Here's how the part is built. I have some questions about the finished solid (model axes, mm). Give positions to 0.01 mm unless a question says otherwise; leave off trailing zeros. Order: outer loops, then holes, each group sorted by start corner. A loop starts at its lowest first (then second) coordinate and runs counter-clockwise, first axis right, second up.
from build123d import *

# Parameters (mm, degrees)
SKETCH1_R           = 4.5
BOSS_EXTRUDE1_DEPTH = 3
SKETCH3_R           = 1.5
CUT_EXTRUDE1_DEPTH  = 10


with BuildPart() as part:
    # Sketch1 → Boss-Extrude1 (new body)
    with BuildSketch(Plane(origin=(0, 0, 0), x_dir=(0, 0, -1), z_dir=(1, 0, 0))):
        with BuildLine():
            Line((0.169822647, 50), (0.169822647, -50))
            ThreePointArc((0.169822647, -50), (-14.830177353, -65), (-29.830177353, -50))
            Line((-29.830177353, -50), (-29.830177353, 50))
            ThreePointArc((-29.830177353, 50), (-14.830177353, 65), (0.169822647, 50))
        make_face()
        with Locations((-14.830177353, -50)):
            Circle(SKETCH1_R, mode=Mode.SUBTRACT)
    extrude(amount=BOSS_EXTRUDE1_DEPTH)

    # Sketch3 → Cut-Extrude1 (cut)
    with BuildSketch(Plane(origin=(3, 0, 0), x_dir=(0, 0, -1), z_dir=(1, 0, 0))):
        with Locations((-14.830177353, 50)):
            Circle(SKETCH3_R)
    extrude(amount=-CUT_EXTRUDE1_DEPTH, mode=Mode.SUBTRACT)


solid = part.part
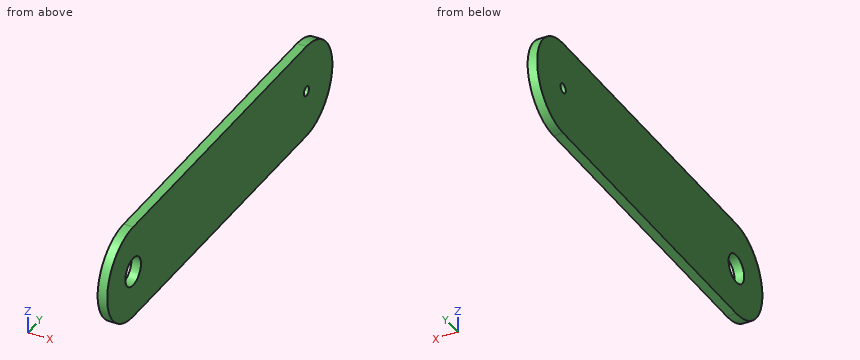
Q1. If we section it at A-A on x = 1: List the corners of the cut face in (y, z) for me, plus the area to 3 significant figures.
Filled sheet:
outline: (-50, -0.17) - (50, -0.17) arc R15 ccw to (50, 29.83) - (-50, 29.83) arc R15 ccw to start; hole circle Ø9 at (-50, 14.83); hole circle Ø3 at (50, 14.83)
area: 3,640 mm2
Q2. I need wall thicknesses on L1, parallel to Z at x = 0.4, y = -48.5; L2, parallel to Y at x = 0.6, z = 16.75; L3, parallel to Z at x = 0.35, y = -54. Which ranges of each line are inside material? Lowest first, please.
Filled sheet:
L1: z = -0.17 to 10.59, 19.07 to 29.83
L2: y = -64.88 to -54.07, -45.93 to 64.88
L3: z = 0.37 to 12.77, 16.89 to 29.29
Q3. I'm going to push a flat-ended pin straight in: P1, Ø1.5, axis at x = 0.5, z = 8, coming from the +Y side. Where does the tip first touch, or does it pass through?
Filled sheet:
P1: stops at y = 63.71
Q4. If we section it at C-C on y = 53.5: List the corners of the cut face in (x, z) for me, plus the area to 3 significant figures.
Filled sheet:
outline: (0, 0.24) - (3, 0.24) - (3, 29.42) - (0, 29.42) - close
area: 87.5 mm2
Q5. If we section it at B-B on z = 8.5: List the corners of the cut face in (x, y) for me.
Filled sheet:
outline: (0, -63.6) - (3, -63.6) - (3, 63.6) - (0, 63.6) - close
